from build123d import *

# Parameters (mm, degrees)
SKETCH1_W           = 6
SKETCH1_H           = 45
BOSS_EXTRUDE1_DEPTH = 20
SKETCH2_R           = 1.5
CUT_EXTRUDE2_DEPTH  = 7


with BuildPart() as part:
    # Sketch1 → Boss-Extrude1 (new body)
    with BuildSketch(Plane.XY):
        with Locations((-10, 0)):
            Rectangle(SKETCH1_W, SKETCH1_H)
    extrude(amount=BOSS_EXTRUDE1_DEPTH)

    # Sketch2 → Cut-Extrude2 (cut, through all)
    with BuildSketch(Plane.ZY.offset(13)):
        with Locations((13, -18.5)):
            Circle(SKETCH2_R)
        with Locations((13, 18.5)):
            Circle(SKETCH2_R)
    extrude(amount=-CUT_EXTRUDE2_DEPTH, mode=Mode.SUBTRACT)


solid = part.part
Read the model definition and answer for the solid it produces. Units are mm, in the model's axes. Round coordinates to 2 decimals unless told otherwise and drop trailing zeros. Loops run counter-clockwise (first coordinate to the right, second up) from the corner with the lowest first, then second, coordinate; pieces in that order, holes last.
Q1. Section C-C on x = -7.65 is taken. Write down the section's boundary in (y, z), and give its area (3 significant figures).
Q2. Section B-B on y = -18.5 is taken. Write down the section's boundary in (x, z), and give its area (3 significant figures).
Q3. Determine the mould class of faces 1 (the face through (-10.04, -17.49, 11.89)), 2 (the face through (-10, 0, 20)), 3 (the face through (-10, -22.5, 10)) for opening direction Z: released by +Z, released by -Z, zero draft, split by the parting line, or undercut.
Q4. Consider probe 1 along Y at (x, z) = (-10.15, 13). Determine where the line is inside the solid, lowest interval first.
Q5. Section A-A on z = 13 is taken. Write down the section's boundary in (x, y).
Output:
1. outline: (-22.5, 0) - (22.5, 0) - (22.5, 20) - (-22.5, 20) - close; hole circle Ø3 at (-18.5, 13); hole circle Ø3 at (18.5, 13)
1. area: 886 mm2
2. outline: (-13, 0) - (-7, 0) - (-7, 11.5) - (-13, 11.5) - close; (-13, 14.5) - (-7, 14.5) - (-7, 20) - (-13, 20) - close
2. area: 102 mm2
3. face 1: undercut
3. face 2: released by +Z
3. face 3: zero draft
4. probe 1: y = -22.5 to -20, -17 to 17, 20 to 22.5
5. outline: (-13, -22.5) - (-7, -22.5) - (-7, -20) - (-13, -20) - close; (-13, -17) - (-7, -17) - (-7, 17) - (-13, 17) - close; (-13, 20) - (-7, 20) - (-7, 22.5) - (-13, 22.5) - close
